Here's the drawing with two shaded views (mm, measured from the low corner). I have some questions. Give positions to 0.01 mm unless a question says otherwise; leave off trailing zeros. Loops run counter-clockwise (first coordinate to the right, second up) from the corner with the lowest first, then second, coordinate; pieces in that order, holes last. Notation, with made-up numbers: (-30.5, 32) - (25.5, 32) arc R26 ccw to (25.5, 55) - close; hole circle Ø8 at (77.5, 52). An arc over 180 degrees is marked (long way). Use a Markdown table: item, result. Add a question column.
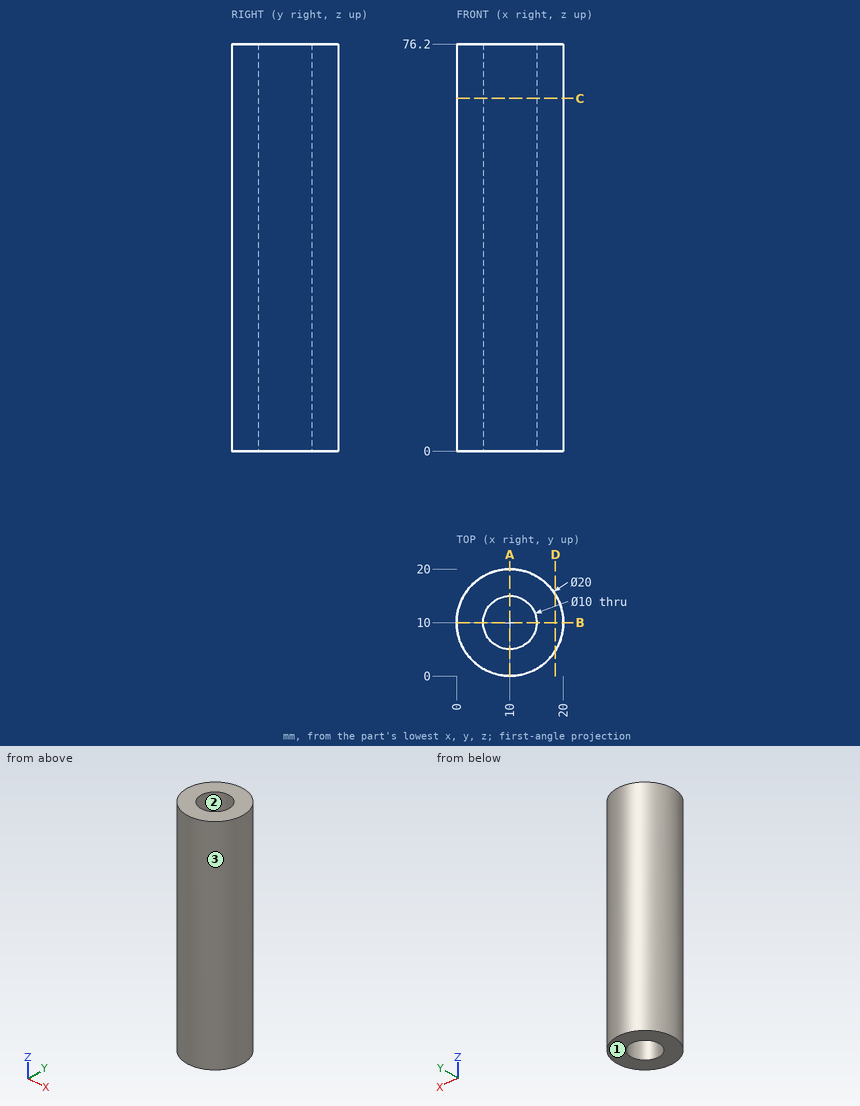
1. Suppose I cut it at D-D (x = 18.5). List the corners of the cut face in (y, z) for me.
2. Suppose I cut it at C-C (z = 66). List the corners of the cut face in (x, y) for me.
3. Please list where these lines run through material, in increasing order: line 1 along Y through (x, z) = (10, 19); line 2 along X through (y, z) = (6, 45). Write a range as [from, to].
4. Will these pins go through, and if not, where does the flat tip stop? P1, Ø4, axis at x = 15, z = 55, coming from the +Y side; P2, Ø10, axis at x = 3.5, z = 41, coming from the -Y side; P3, Ø2, axis at y = 9, z = 8.5, coming from the -X side; P4, Ø6, axis at y = 15, z = 22, coming from the +X side.
5. If we mould it in two halves opening along Y, with no side actions, what happens to the marked faces 1, 2 and 3? For each: released by +Y, released by -Y, zero draft, split by the parting line, or undercut.
6. Suppose I cut it at A-A (x = 10). List the corners of the cut face in (y, z) for me, and give its area (3 significant figures).
Results below:
| question | item | result |
|---|---|---|
| 1 | outline | (4.73, 0) - (15.27, 0) - (15.27, 76.2) - (4.73, 76.2) - close |
| 2 | outline | circle Ø20 at (10, 10); hole circle Ø10 at (10, 10) |
| 3 | line 1 | [0, 5], [15, 20] |
| 3 | line 2 | [0.83, 7], [13, 19.17] |
| 4 | P1 | y = 19.54 |
| 4 | P2 | y = 0.11 |
| 4 | P3 | x = 0 |
| 4 | P4 | x = 19.8 |
| 5 | face 1 | zero draft |
| 5 | face 2 | undercut |
| 5 | face 3 | split by the parting line |
| 6 | outline | (0, 0) - (5, 0) - (5, 76.2) - (0, 76.2) - close; (15, 0) - (20, 0) - (20, 76.2) - (15, 76.2) - close |
| 6 | area | 762 mm² |
